Work out the finished part from the listing and answer in its coordinate system (mm). A direction names the side the tool comes from. Round coordinates to 2 decimals unless told otherwise and drop trailing zeros. Write each loop counter-clockwise with the first axis right and the second up, starting at its lowest first coordinate (ties: lowest second). Pieces come first, ordered by that corner, then holes. Notation, with made-up numbers: M -2,18.25 L 13,18.25 A8 ccw 13,29.25 Z; hole C 10,63 d11. An arc over 180 degrees is marked long. Answer in a Markdown table with one row per item.
Autodesk Inventor part; units mm, degrees
ref_plane "YZ Plane" through (0, 0, 0) normal (1, 0, 0) x (0, 1, 0)
ref_plane "XZ Plane" through (0, 0, 0) normal (0, 1, 0) x (-1, 0, 0)
ref_plane "XY Plane" through (0, 0, 0) normal (0, 0, 1) x (1, 0, 0)
sketch "Эскиз1" plane through (0, 0, 0) normal (0, 0, 1) x (1, 0, 0)
  line L0 (-7, -3.5) -> (7, -3.5) construction
  line L1 (7, -3.5) -> (7, 3.5)
  line L2 (7, 3.5) -> (-7, 3.5)
  line L3 (-7, 3.5) -> (-7, -3.5)
  line L4 (-7, -3.5) -> (7, 3.5) construction
  line L5 (7, -3.5) -> (-7, 3.5) construction
  line L6 (0, -3.5) -> (0, -12.5) construction
  line L7 (-7, -3.5) -> (-3.289, -13.697)
  line L8 (7, -3.5) -> (3.289, -13.697)
  arc A0 (-3.289, -13.697) -> (3.289, -13.697) centre (0, -12.5) ccw
  point P0 (0, 0)
  point P1 (0, 0)
  point P2 (0, 0)
  point P3 (0, 0)
  dimension "d0" = 14
  dimension "d1" = 7
  dimension "d4" = 9
  dimension "d5" = 3.5
extrude "Выдавливание1" add sketch "Эскиз1" along normal blind 1.5
sketch "Эскиз4" plane through (0, 0, 1.5) normal (0, 0, 1) x (1, 0, 0)
  line L0 (7, 3.5) -> (-7, 3.5)
  line L1 (7, -3.5) -> (7, 3.5)
  line L2 (-7, 3.5) -> (-7, -3.5)
  line L3 (-7, -3.5) -> (7, -3.5)
  point P0 (0, 0)
extrude "Выдавливание6" add sketch "Эскиз4" along normal blind 3.4
sketch "Эскиз2" plane through (0, 0, 1.5) normal (0, 0, 1) x (1, 0, 0)
  arc A0 (-3.289, -13.697) -> (3.289, -13.697) centre (0, -12.5) ccw construction
  circle A1 centre (0, -12.5) radius 1.25
  point P0 (0, 0)
  dimension "d8" = 2.5
extrude "Выдавливание9" add sketch "Эскиз2" along normal blind 5
fillet "Сопряжение1" radius 3.5 2 edges at (7, 3.5, 2.45) (-7, 3.5, 2.45)
sketch "Эскиз5" plane through (0, 0, 4.9) normal (0, 0, 1) x (1, 0, 0)
  circle A0 centre (0, -9.5) radius 1.5 construction
  line L0 (7, -3.5) -> (-7, -3.5) construction
  line L1 (0, -3.5) -> (0, 3.5) construction
  line L2 (-7, 3.5) -> (7, 3.5) construction
  circle A1 centre (3.5, 0) radius 0.5
  line L3 (3.5, 3.5) -> (3.5, 0) construction
  line L4 (3.5, 0) -> (0, 0) construction
  circle A2 centre (-3.5, 0) radius 0.5
  dimension "d34" = 1
hole "Отверстие1" at (-3.5, 0, 4.9) at (3.5, 0, 4.9) direction (0, 0, -1) diameter 1 end through all countersink diameter 1.5 countersink angle 90
properties part number "переходник"
1. Consider line 1 along X through (y, z) = (0, 1.75); line 2 along Y through (x, z) = (0, 4.25); line 3 along Y through (x, z) = (3.5, 1.85). Determine where each line is inside the solid, lowest interval first. Write a range as from..to.
Calculated:
| item | result |
|---|---|
| line 1 | x = -7..-4, -3..3, 4..7 |
| line 2 | y = -13.75..-11.25, -3.5..3.5 |
| line 3 | y = -3.5..-0.5, 0.5..3.5 |
2. The part is cut by section B-B (x = 0). Determine the outline of the cut face in (y, z), plus the area to 4 significant figures.
Calculated:
| item | result |
|---|---|
| outline | M -16,0 L 3.5,0 L 3.5,4.9 L -3.5,4.9 L -3.5,1.5 L -11.25,1.5 L -11.25,6.5 L -13.75,6.5 L -13.75,1.5 L -16,1.5 Z |
| area | 65.55 mm² |
3. Given pin 1 (1 mm diameter, centred on x = 4, y = -1.5, fed in from -Z); pin 2 (2 mm diameter, centred on y = -13.5, z = 2, fed in from -X); pin 3 (2 mm diameter, centred on x = 5, y = 0, fed in from +Z); pin 4 (1.7 mm diameter, centred on x = -2.5, z = 2.5, fed in from -Y), each flat-ended and moving along its own axis, determine where each tip first touches the part or whether it passes through.
Calculated:
| item | result |
|---|---|
| pin 1 | stops at z = 0 |
| pin 2 | stops at x = -3.68 |
| pin 3 | stops at z = 4.9 |
| pin 4 | stops at y = -3.5 |
4. The part is cut by section D-D (z = 6.25). Determine the outline of the cut face in (x, y).
Calculated:
| item | result |
|---|---|
| outline | C 0,-12.5 d2.5 |
5. The part is cut by section C-C (y = -12.5). Determine the outline of the cut face in (x, z), plus the area to 3 significant figures.
Calculated:
| item | result |
|---|---|
| outline | M -3.72,0 L 3.72,0 L 3.72,1.5 L 1.25,1.5 L 1.25,6.5 L -1.25,6.5 L -1.25,1.5 L -3.72,1.5 Z |
| area | 23.7 mm² |
6. The part is cut by section A-A (z = 3.25). Determine the outline of the cut face in (x, y).
Calculated:
| item | result |
|---|---|
| outline | M -7,-3.5 L 7,-3.5 L 7,0 A3.5 ccw 3.5,3.5 L -3.5,3.5 A3.5 ccw -7,0 Z; C 0,-12.5 d2.5; hole C -3.5,0 d1; hole C 3.5,0 d1 |
7. A tool of negligible diameter and unlimited length cuts with its end or side. For faces 1 (the flat face through (0, 0, 4.9)), 2 (the cylindrical face through (-0.16, -13.74, 3.96)), 3 (the flat face through (7, -2, 2)), from which of +Z, -Z, +X, -X, +Y, -Y can it reach the whole face along a straight path? Write none if from no direction.
Calculated:
| item | result |
|---|---|
| face 1 | +Z, +X, -X, +Y |
| face 2 | +Z |
| face 3 | +Z, -Z, +X, +Y, -Y |
8. Determine the mould class of faces 4 (the cylindrical face through (-5.95, 2.5, 2.48)), 5 (the cylindrical face through (3, 0, 2)), 6 (the flat face through (0, -8, 1.5)) for opening direction X: released by +X, released by -X, zero draft, split by the parting line, or undercut.
Calculated:
| item | result |
|---|---|
| face 4 | released by -X |
| face 5 | undercut |
| face 6 | zero draft |
